```python
from build123d import *

# Parameters (mm, degrees)
SKETCH_R     = 1.6
PAD_DEPTH    = 6
SKETCH001_R  = 1.6
POCKET_DEPTH = 8.001
FILLET_R     = 3


with BuildPart() as part:
    # Sketch → Pad (new body, symmetric)
    with BuildSketch(Plane.XY):
        Polygon((1.514719, 20), (18.828427, 20), (18.828427, 10), (6.828427, 10), (2.828427, 10), (0, 7.171573), (0, -7.171573), (2.828427, -10), (6.828427, -10), (18.828427, -10), (18.828427, -20), (1.514719, -20), (-8, -10.485281), (-8, 10.485281), align=None)
        with Locations((12.828427, 14)):
            Circle(SKETCH_R, mode=Mode.SUBTRACT)
        with Locations((12.828427, -14)):
            Circle(SKETCH_R, mode=Mode.SUBTRACT)
    extrude(amount=PAD_DEPTH, both=True)

    # Sketch001 → Pocket (cut, through all)
    with BuildSketch(Plane.YZ):
        Circle(SKETCH001_R)
    extrude(amount=-POCKET_DEPTH, mode=Mode.SUBTRACT)

    # Fillet
    fillet_edges = [part.edges().sort_by_distance(p)[0] for p in [
        (18.828427, -20, 0),
        (18.828427, -10, 0),
        (18.828427, 10, 0),
        (18.828427, 20, 0),
        (1.514719, -20, 0),
        (-8, -10.485281, 0),
        (-8, 10.485281, 0),
        (1.514719, 20, 0),
        (2.828427, 10, 0),
        (0, 7.171573, 0),
        (0, -7.171573, 0),
        (2.828427, -10, 0),
    ]]
    fillet(fillet_edges, radius=FILLET_R)


solid = part.part
```
Geometry check sheet. Reference: the model listing, model coordinates, mm. A direction names the side the tool comes from. Coordinates: 2 decimals unless noted, no trailing zeros. Loops run counter-clockwise (first coordinate to the right, second up) from the corner with the lowest first, then second, coordinate; pieces in that order, holes last.
Item 1: Access from +Z, -Z, +X, -X, +Y, -Y to the whole of each face (thin tool, end or side, straight path). Record for faces 1 (the face through (9, 20, 0)), 2 (the face through (0.235, 7.092, -0.084)).
Item 2: Go/stop test with flat-tipped pins: pin 1 Ø1 at (y, z) = (15, 4.5) entering from -X; pin 2 Ø6 at (y, z) = (-9.5, -2) entering from +X. Record where each tip stops, or that it passes through.
Item 3: Release check for a two-part mould opening along Y. For faces 3 (the face through (10, -10, 0)), 4 (the face through (17.97, 10.9, -0.08)), 5 (the face through (17.93, -19.14, 0.08)), 6 (the face through (18.828, -15, 0)) record: released by +Y, released by -Y, zero draft, split by the parting line, or undercut.
Item 4: Thickness scan on line 1 (Y direction, x = 10.5, z = 2.75); line 2 (Y direction, x = 13.25, z = 2.5); line 3 (Z direction, x = -5.75, y = 0). Record the ranges inside material, lowest first.
Item 5: Sectioned sample at C-C, the plane y = 0. Record the boundary of the cut face in (x, z), then the cut area to 3 significant figures.
Item 6: Sectioned sample at B-B, the plane x = 10.5. Record the boundary of the cut face in (y, z).
Item 7: Sectioned sample at A-A, the plane z = 0. Count the separate pieces of the cut face and the enclosed holes in it, then the cut area to 3 significant figures.
Item 8: Sectioned sample at D-D, the plane y = 5. Record the boundary of the cut face in (x, z), then the cut area to 3 significant figures.
Check result:
1. face 1: +Z, -Z, +X, -X, +Y
1. face 2: +Z, -Z, +X
2. pin 1: stops at x = -3.99
2. pin 2: stops at x = 18.79
3. face 3: undercut
3. face 4: undercut
3. face 5: released by -Y
3. face 6: zero draft
4. line 1: y = -20 to -10, 10 to 20
4. line 2: y = -20 to -15.54, -12.46 to -10, 10 to 12.46, 15.54 to 20
4. line 3: z = -6 to -1.6, 1.6 to 6
5. outline: (-8, -6) - (0, -6) - (0, -1.6) - (-8, -1.6) - close; (-8, 1.6) - (0, 1.6) - (0, 6) - (-8, 6) - close
5. area: 70.4 mm2
6. outline: (-20, -6) - (-10, -6) - (-10, 6) - (-20, 6) - close; (10, -6) - (20, -6) - (20, 6) - (10, 6) - close
7. separate pieces: 2
7. enclosed holes: 2
7. area: 565 mm2
8. outline: (-8, -6) - (0, -6) - (0, 6) - (-8, 6) - close
8. area: 96.0 mm2
